```python
from build123d import *

# Parameters (mm, degrees)
F0_W      = 29
F0_H      = 16.5
F1_DEPTH  = 38.5
F2_T      = -2
F3_DEPTH  = 2.25
F4_SIZE   = 2
F5_SIZE   = 2
F6_SIZE   = 2
F7_SIZE   = 2
F8_SIZE   = 2
F9_SIZE   = 0.99999
F11_DEPTH = 16.501
F12_SIZE  = 2
F13_SIZE  = 2
F14_W     = 12.5
F14_H     = 2.3482141793
F15_DEPTH = 2
F16_R     = 2
F17_DEPTH = 2.001
F18_W     = 7.1378413203
F18_H     = 7.25
F18_R     = 1.1
F19_DEPTH = 4.35


# Not quite as in the source:
# - a fillet or chamfer is up to 0.001 mm smaller than in the source, because OpenCascade refuses the exact size


with BuildPart() as f1:
    # F0 (on Top) → F1 (new body)
    with BuildSketch(Plane.XY):
        with Locations((14.5, 8.25)):
            Rectangle(F0_W, F0_H)
    extrude(amount=F1_DEPTH)

    # F2
    f2_openings = [f1.faces().sort_by_distance(p)[0] for p in [
        (14.5, 8.25, 38.5),
    ]]
    offset(amount=F2_T, openings=f2_openings)

    # F3 (add): a face of the model
    f3_faces = [f1.faces().sort_by_distance(p)[0] for p in [
        (14.5, 8.25, 2),
    ]]
    extrude(f3_faces, amount=F3_DEPTH)

    # F4
    f4_edges = [f1.edges().sort_by_distance(p)[0] for p in [
        (0, 0, 19.25),
    ]]
    chamfer(f4_edges, length=F4_SIZE)

    # F5
    f5_edges = [f1.edges().sort_by_distance(p)[0] for p in [
        (0, 16.5, 19.25),
        (29, 0, 19.25),
    ]]
    chamfer(f5_edges, length=F5_SIZE)

    # F6
    f6_edges = [f1.edges().sort_by_distance(p)[0] for p in [
        (29, 16.5, 19.25),
    ]]
    chamfer(f6_edges, length=F6_SIZE)

    # F7
    f7_edges = [f1.edges().sort_by_distance(p)[0] for p in [
        (14.5, 0, 0),
    ]]
    chamfer(f7_edges, length=F7_SIZE)

    # F8
    f8_edges = [f1.edges().sort_by_distance(p)[0] for p in [
        (14.5, 16.5, 0),
    ]]
    chamfer(f8_edges, length=F8_SIZE)

    # F9 (size 1 in the source; OpenCascade refuses exactly that, so slightly less here)
    f9_edges = [f1.edges().sort_by_distance(p)[0] for p in [
        (14.5, 14.5, 38.5),
        (2, 8.25, 38.5),
        (14.5, 2, 38.5),
        (27, 8.25, 38.5),
    ]]
    chamfer(f9_edges, length=F9_SIZE)

    # F10 (on face) → F11 (cut, through all)
    with BuildSketch(Plane(origin=(0, 16.5, 0), x_dir=(-1, 0, 0), z_dir=(0, 1, 0))):
        Polygon((-16.345, 12.834), (-22.516, 8.664), (-22.516, 4.94), (-5.445, 4.94), (-5.445, 8.664), (-11.616, 12.834), align=None)
    extrude(amount=-F11_DEPTH, mode=Mode.SUBTRACT)

    # F12
    f12_edges = [f1.edges().sort_by_distance(p)[0] for p in [
        (0, 8.25, 0),
    ]]
    chamfer(f12_edges, length=F12_SIZE)

    # F13
    f13_edges = [f1.edges().sort_by_distance(p)[0] for p in [
        (29, 8.25, 0),
    ]]
    chamfer(f13_edges, length=F13_SIZE)

    # F14 (on face) → F15 (cut, through all)
    with BuildSketch(Plane(origin=(0, 0, 0), x_dir=(0, -1, 0), z_dir=(-1, 0, 0))):
        with BuildLine():
            ThreePointArc((-14.5, 28.5), (-8.25, 34.75), (-2, 28.5))
            Line((-2, 28.5), (-2, 38.5))
            Line((-2, 38.5), (-14.5, 38.5))
            Line((-14.5, 38.5), (-14.5, 28.5))
        make_face()
        with Locations((-8.25, 39.6741070896)):
            Rectangle(F14_W, F14_H)
        with BuildLine():
            Line((-14.5, 28.5), (-2, 28.5))
            ThreePointArc((-2, 28.5), (-8.25, 34.75), (-14.5, 28.5))
        make_face()
        with BuildLine():
            ThreePointArc((-11.8148919341, 23.3663808577), (-8.6306663931, 22.2616033232), (-5.335738673, 22.9710235198))
            ThreePointArc((-5.335738673, 22.9710235198), (-5.3356417901, 22.985511616), (-5.3356094956, 23))
            ThreePointArc((-5.3356094956, 23), (-8.4021264241, 26.2448164759), (-11.8148919341, 23.3663808577))
        make_face()
        with BuildLine():
            ThreePointArc((-11.8148919341, 23.3663808577), (-8.7835560201, 19.7560337281), (-5.335738673, 22.9710235198))
            ThreePointArc((-5.335738673, 22.9710235198), (-8.6306663931, 22.2616033232), (-11.8148919341, 23.3663808577))
        make_face()
        with BuildLine():
            ThreePointArc((-5.335738673, 22.9710235198), (-2.8985220129, 25.2713496081), (-2, 28.5))
            Line((-2, 28.5), (-14.5, 28.5))
            ThreePointArc((-14.5, 28.5), (-13.7881889905, 25.6032841517), (-11.8148919341, 23.3663808577))
            ThreePointArc((-11.8148919341, 23.3663808577), (-8.4021264241, 26.2448164759), (-5.3356094956, 23))
            ThreePointArc((-5.3356094956, 23), (-5.3356417901, 22.985511616), (-5.335738673, 22.9710235198))
        make_face()
    extrude(amount=-F15_DEPTH, mode=Mode.SUBTRACT)

    # F16 (on face) → F17 (cut, through all)
    with BuildSketch(Plane(origin=(27, 0, 0), x_dir=(0, -1, 0), z_dir=(-1, 0, 0))):
        with Locations((-8.5856094956, 23)):
            Circle(F16_R)
    extrude(amount=-F17_DEPTH, mode=Mode.SUBTRACT)

    # F18 (on face) → F19 (join)
    with BuildSketch(Plane(origin=(0, 0, 0), x_dir=(0, -1, 0), z_dir=(-1, 0, 0))):
        with Locations((-8.0489206601, 7.875)):
            Rectangle(F18_W, F18_H)
        with Locations((-8.25, 9)):
            Circle(F18_R, mode=Mode.SUBTRACT)
    extrude(amount=F19_DEPTH)


solid = f1.part
```
Read the model definition and answer for the solid it produces. Units are mm, in the model's axes. A direction names the side the tool comes from. Coordinates: 2 decimals unless noted, no trailing zeros. Loops run counter-clockwise (first coordinate to the right, second up) from the corner with the lowest first, then second, coordinate; pieces in that order, holes last. Notation, with made-up numbers: (53, 14.5) -> (66, 14.5) arc R21 cw to (66, 52.5) -> close; hole circle Ø2 at (55, 77). An arc over 180 degrees is marked (long way). Return JSON: item names as keys, results as strings.
Item 1: Find section A-A (x = 17). Determine the outline of the cut face in (y, z), plus the area to 3 significant figures.
Answers:
{"outline": "(0, 2) -> (2, 0) -> (14.5, 0) -> (16.5, 2) -> (16.5, 4.94) -> (14.5, 4.94) -> (14.5, 4.25) -> (2, 4.25) -> (2, 4.94) -> (0, 4.94) -> close; (0, 12.39) -> (2, 12.39) -> (2, 37.5) -> (1, 38.5) -> (0, 38.5) -> close; (14.5, 12.39) -> (16.5, 12.39) -> (16.5, 38.5) -> (15.5, 38.5) -> (14.5, 37.5) -> close", "area": "172 mm2"}
Item 2: For faces 1 (the flat face through (22.516, 16, 7)), 2 (the flat face through (14, 8, 4.25)), 3 (the cylindrical face through (0.986, 13.808, 25.641)), 4 (the flat face through (-2, 8, 4.25)), determine the directions among +Z, -Z, +X, -X, +Y, -Y from which every point of the face is accessible in a straight line to the end or side of a thin tool.
Answers:
{"face 1": "+Y, -Y", "face 2": "+Z", "face 3": "+Z, -X", "face 4": "-Z, -X, +Y, -Y"}
Item 3: Find section C-C (z = 9.5). Determine the outline of the cut face in (x, y).
Answers:
{"outline": "(-4.35, 4.48) -> (0, 4.48) -> (0, 2) -> (2, 0) -> (6.68, 0) -> (6.68, 2) -> (2, 2) -> (2, 14.5) -> (6.68, 14.5) -> (6.68, 16.5) -> (2, 16.5) -> (0, 14.5) -> (0, 11.62) -> (-4.35, 11.62) -> (-4.35, 9.23) -> (0, 9.23) -> (0, 7.27) -> (-4.35, 7.27) -> close; (21.28, 0) -> (27, 0) -> (29, 2) -> (29, 14.5) -> (27, 16.5) -> (21.28, 16.5) -> (21.28, 14.5) -> (27, 14.5) -> (27, 2) -> (21.28, 2) -> close"}
Item 4: Flat-ended cylindrical pins translate along their axes: P1, Ø0.6, axis at y = 15.5, z = 7, coming from the +X side; P2, Ø5, axis at x = -3, y = 9.5, coming from the -Z side; P3, Ø3.5, axis at x = -1, z = 8.5, coming from the -Y side. Find the tip coordinate at first contact, or state that the pin passes through.
Answers:
{"P1": "stops at x = 28.3", "P2": "stops at z = 4.25", "P3": "stops at y = 1.25"}
Item 5: For a pull along Z with two mould halves and no side action, classify faces 5 (the flat face through (14.3, 1.5, 38)), 6 (the flat face through (-4.35, 8, 7)), 7 (the flat face through (5.445, 1, 7)), 8 (the flat face through (14.3, 15.5, 1)) as +Z half, -Z half, draft (parallel to the pull), parting line (faces both ways), or undercut.
Answers:
{"face 5": "+Z half", "face 6": "draft", "face 7": "undercut", "face 8": "-Z half"}
Item 6: Find section D-D (x = 3). Determine the outline of the cut face in (y, z).
Answers:
{"outline": "(0, 2) -> (2, 0) -> (14.5, 0) -> (16.5, 2) -> (16.5, 38.5) -> (15.5, 38.5) -> (14.5, 37.5) -> (14.5, 4.25) -> (2, 4.25) -> (2, 37.5) -> (1, 38.5) -> (0, 38.5) -> close"}
Item 7: Find section B-B (y = 8.25). Determine the outline of the cut face in (x, z), plus the area to 3 significant figures.
Answers:
{"outline": "(-4.35, 4.25) -> (0, 4.25) -> (0, 2) -> (2, 0) -> (27, 0) -> (29, 2) -> (29, 21.03) -> (27, 21.03) -> (27, 4.25) -> (2, 4.25) -> (2, 19.77) -> (0, 19.77) -> (0, 11.5) -> (-4.35, 11.5) -> (-4.35, 10.1) -> (0, 10.1) -> (0, 7.9) -> (-4.35, 7.9) -> close; (27, 24.97) -> (29, 24.97) -> (29, 38.5) -> (28, 38.5) -> (27, 37.5) -> close", "area": "232 mm2"}
Item 8: Find the intervals of material crossed by probe 1 along X at (y, z) = (10, 11); probe 2 along Y at (x, z) = (11, 12.5); probe 3 along Z at (x, y) = (-3, 8.25), in increasing order.
Answers:
{"probe 1": "x = -4.35 to 2, 27 to 29", "probe 2": "y = 0 to 2, 14.5 to 16.5", "probe 3": "z = 4.25 to 7.9, 10.1 to 11.5"}
